```python
from build123d import *

# Parameters (mm, degrees)
F0_R      = 57.7881585004
F1_DEPTH  = 12.5
F2_W      = 44.1803280264
F2_H      = 27.6844277978
F4_DEPTH  = 37.5
F3_W      = 67.8
F3_H      = 7.7
F5_DEPTH  = 12.5
F6_T      = -2.5
F7_W      = 50.2489116043
F7_H      = 8.9359693229
F8_DEPTH  = 50
F10_R     = 10.5252112218
F11_DEPTH = 50
F9_R      = 8.9119309546
F12_DEPTH = 50


with BuildPart() as f1:
    # F0 (on Front) → F1 (new body, symmetric)
    with BuildSketch(Plane.XZ):
        with Locations((2.5819686707, 0)):
            Circle(F0_R)
    extrude(amount=F1_DEPTH, both=True)

    # F2 (on face) → F4 (join, symmetric)
    with BuildSketch(Plane.XZ.offset(12.5)):
        with Locations((6.0245888308, 13.8422138989)):
            Rectangle(F2_W, F2_H)
    extrude(amount=F4_DEPTH, both=True)

    # F3 (on face) → F5 (cut, symmetric)
    with BuildSketch(Plane.XZ.offset(12.5)):
        with Locations((2.5539135873, -26.7082657456)):
            Rectangle(F3_W, F3_H)
    extrude(amount=F5_DEPTH, both=True, mode=Mode.SUBTRACT)

    # F6
    f6_openings = [f1.faces().sort_by_distance(p)[0] for p in [
        (6.024589, -50, 13.842214),
    ]]
    offset(amount=F6_T, openings=f6_openings, kind=Kind.INTERSECTION)

    # F7 (on face) → F8 (join)
    with BuildSketch(Plane(origin=(0, 12.5, 0), x_dir=(-1, 0, 0), z_dir=(0, 1, 0))):
        with Locations((-0.5627823994, 40.6393650919)):
            Rectangle(F7_W, F7_H)
    extrude(amount=F8_DEPTH)

    # F10 (on face) → F11 (join)
    with BuildSketch(Plane(origin=(0, 12.5, 0), x_dir=(-1, 0, 0), z_dir=(0, 1, 0))):
        with Locations((-32.1311503649, -33.1352464855)):
            Circle(F10_R)
    extrude(amount=F11_DEPTH)

    # F9 (on face) → F12 (join)
    with BuildSketch(Plane(origin=(0, 12.5, 0), x_dir=(-1, 0, 0), z_dir=(0, 1, 0))):
        with Locations((28.9754085243, -35.4303270578)):
            Circle(F9_R)
    extrude(amount=F12_DEPTH)


solid = f1.part
```
Design review of the part built by this model. Coordinates are the model's own, in mm. A direction names the side the tool comes from. Round coordinates to 2 decimals unless told otherwise and drop trailing zeros. Order: outer loops, then holes, each group sorted by start corner. A loop starts at its lowest first (then second) coordinate and runs counter-clockwise, first axis right, second up. Notation, with made-up numbers: M 19.25,5 L 63.25,5 A26 ccw 63.25,24 Z; hole C 12.5,32.25 d3. An arc over 180 degrees is marked long. Put each result on its own line as item: value.
Q1. Insertion check: pin 1 Ø4 at (x, y) = (13, 18.5) entering from -Z; pin 2 Ø22 at (x, z) = (-2, 12.5) entering from +Y; pin 3 Ø4 at (x, z) = (-28.5, 41.5) entering from -Y. Each pin has a flat end and moves straight along its axis. Give the tip position at first contact, or say it passes through.
Reported:
pin 1: z = 0
pin 2: y = 25
pin 3: y = -12.5
Q2. Consider section B-B (z = -5.5). State the section outline as (x, y) points, and give its area (3 significant figures).
Reported:
outline: M -54.94,-12.5 L 60.11,-12.5 L 60.11,12.5 L -54.94,12.5 Z; hole M -52.43,-10 L 57.6,-10 L 57.6,10 L -52.43,10 Z
area: 676 mm²
Q3. To check wall thickness, follow line 1 (Z direction, x = -11, y = -28.5); line 2 (X direction, y = -24.5, z = 10); line 3 (Y direction, x = -19, z = -42.5). State the ranges of each line that lie inside material, in increasing order.
Reported:
line 1: 0 to 2.5, 25.18 to 27.68
line 2: -16.07 to -13.57, 25.61 to 28.11
line 3: -12.5 to -10, 10 to 12.5
Q4. Consider section A-A (y = -20). State the section outline as (x, z) points.
Reported:
outline: M -16.07,0 L 28.11,0 L 28.11,27.68 L -16.07,27.68 Z; hole M -13.57,2.5 L 25.61,2.5 L 25.61,25.18 L -13.57,25.18 Z
Q5. Machinability: for faces 1 (the face through (-21.9, 37.15, -40.85)), 2 (the face through (-16.066, -32, 14)), 3 (the face through (6, 16, 25.184)), 4 (the face through (-33.846, -4, -27)), which of the approach directions +Z, -Z, +X, -X, +Y, -Y give a long, thin tool a straight path to every point of the face, cutting with its end or side? Answer none if there is none.
Reported:
face 1: +Y
face 2: +Z, -Z, -X, -Y
face 3: -Y
face 4: none
Q6. Consider section C-C (y = 48.5). State the section outline as (x, z) points.
Reported:
outline: C -28.98,-35.43 d17.82; M -24.56,36.17 L 25.69,36.17 L 25.69,45.11 L -24.56,45.11 Z; C 32.13,-33.14 d21.05
Q7. Draft analysis for pull direction X (two halves, no side actions). For faces 5 (the face through (-9.945, -0.175, -56.414)), 6 (the face through (-13.566, 16, 14)), 7 (the face through (-29, 62.5, -35)), 8 (the face through (2, 10, 1)), state which applies: released by +X, released by -X, zero draft, split by the parting line, or undercut.
Reported:
face 5: split by the parting line
face 6: undercut
face 7: zero draft
face 8: undercut
